```python
from build123d import *

# Parameters (mm, degrees)
F0_R     = 13.335
F0_R_2   = 9.525
F1_DEPTH = 5.08
F4_DEPTH = 3.556


with BuildPart() as f1:
    # F0 (on Front) → F1 (new body)
    with BuildSketch(Plane.XZ):
        Circle(F0_R)
        Circle(F0_R_2, mode=Mode.SUBTRACT)
    extrude(amount=F1_DEPTH)

    # F3 (on offset) → F4 (join)
    with BuildSketch(Plane.XY.offset(10.16)):
        Polygon((-1.232519, -4.1148), (-1.27, -0.635), (-2.417171, -1.423591), (-2.172425, -1.779626), (-1.510733, -1.324764), (-1.510733, -4.1148), (-2.177129, -4.1148), (-2.177129, -4.445), (-0.686343, -4.445), (-0.686343, -4.1148), align=None)
        Polygon((2.006021, -1.027081), (0.762, -4.445), (1.27, -4.445), (2.656727, -0.635), (0.513302, -0.635), (0.513302, -1.027081), align=None)
    extrude(amount=F4_DEPTH)


solid = f1.part
```
Geometry check sheet. Reference: the model listing, model coordinates, mm. A direction names the side the tool comes from. Round coordinates to 2 decimals unless told otherwise and drop trailing zeros. Order: outer loops, then holes, each group sorted by start corner. A loop starts at its lowest first (then second) coordinate and runs counter-clockwise, first axis right, second up. Notation, with made-up numbers: (67.5, -38) - (114.5, -38) arc R23 ccw to (114.5, -27) - close; hole circle Ø9 at (33.5, 43.25). An arc over 180 degrees is marked (long way). Use a Markdown table: item, result. Add a question column.
(1) Material ranges on line 1 along Z through (x, y) = (0, -1.85) (3 decimals); line 2 along Z through (x, y) = (-5.75, -0.45); line 3 along X through (y, z) = (-3.1, -5.5), recorded low to high. Write a range as [from, to].
(2) Sectioned sample at C-C, the plane y = -2.65. Enter the section's corners in (x, z) (3 decimals), and give its area (3 significant figures).
(3) Sectioned sample at A-A, the plane x = 0. Enter the section's corners in (y, z) (3 decimals), and give its area (3 significant figures).
(4) Depth check by flat-ended pin: pin 1 (0.5 mm diameter, centred on x = 1, z = 13.5, fed in from -Y); pin 2 (11.5 mm diameter, centred on x = 0, z = 0, fed in from -Y); pin 3 (3 mm diameter, centred on y = -4, z = 7, fed in from +X). Enter the tip coordinate at first touch or a pass-through.
(5) Release check for a two-part mould opening along Y. For faces 3 (the flat face through (9, 0, -6)), 4 (the flat face through (1.393, -2.712, 13.505)), 5 (the flat face through (9, -5.08, -6)) record: pulls with the +Y half, pulls with the -Y half, needs draft (parallel to the pull), parting line crosses it, or undercut.
(6) Sectioned sample at D-D, the plane x = 11.5. Enter the section's corners in (y, z).
(7) Tool access check on faces 1 (the flat face through (2, -2, 13.716)), 2 (the flat face through (1.954, -2.567, 13.459)). Record the directions out of +Z, -Z, +X, -X, +Y, -Y that give a thin tool (end or side, any length) a straight path to the whole face; none if there is none.
(8) Sectioned sample at B-B, the plane z = 0. Enter the section's corners in (x, y) (3 decimals).
Answers below:
| question | item | result |
|---|---|---|
| 1 | line 1 | [-13.335, -9.525], [9.525, 13.335] |
| 1 | line 2 | [-12.03, -7.59], [7.59, 12.03] |
| 1 | line 3 | [-12.15, -7.78], [7.78, 12.15] |
| 2 | outline | (-1.511, 13.249) arc R13.335 ccw (long way) to (1.923, 13.196) - (1.923, 13.716) - (1.415, 13.716) - (1.415, 13.26) arc R13.335 ccw to (-1.248, 13.276) - (-1.248, 13.716) - (-1.511, 13.716) - close; hole circle Ø19.05 at (0, 0) |
| 2 | area | 274 mm² |
| 3 | outline | (-5.08, -13.335) - (0, -13.335) - (0, -9.525) - (-5.08, -9.525) - close; (-5.08, 9.525) - (0, 9.525) - (0, 13.335) - (-5.08, 13.335) - close |
| 3 | area | 38.7 mm² |
| 4 | pin 1 | y = -5.08 |
| 4 | pin 2 | through |
| 4 | pin 3 | x = 12.15 |
| 5 | face 3 | pulls with the +Y half |
| 5 | face 4 | undercut |
| 5 | face 5 | pulls with the -Y half |
| 6 | outline | (-5.08, -6.75) - (0, -6.75) - (0, 6.75) - (-5.08, 6.75) - close |
| 7 | face 1 | +Z, +X, -X, +Y, -Y |
| 7 | face 2 | +Z, +X, -Y |
| 8 | outline | (-13.335, -5.08) - (-9.525, -5.08) - (-9.525, 0) - (-13.335, 0) - close; (9.525, -5.08) - (13.335, -5.08) - (13.335, 0) - (9.525, 0) - close |
